Part model, mm, in its own coordinate system. A direction names the side the tool comes from. Round coordinates to 2 decimals unless told otherwise and drop trailing zeros. Order: outer loops, then holes, each group sorted by start corner. A loop starts at its lowest first (then second) coordinate and runs counter-clockwise, first axis right, second up. Notation, with made-up numbers: (61.25, -32.5) -> (93.25, -32.5) arc R22 ccw to (93.25, -19.5) -> close; hole circle Ø7 at (15, 71). An arc over 180 degrees is marked (long way). Answer as a JSON object with one key per item and string values. Group by question number.
```python
from build123d import *

# Parameters (mm, degrees)
SKETCH_W        = 120
SKETCH_H        = 100
PAD_DEPTH       = 22
SKETCH001_R     = 4.5
POCKET_DEPTH    = 22.001
POCKET001_DEPTH = 22.001
SKETCH003_R     = 1
POCKET002_DEPTH = 22.001
SKETCH004_R     = 10
POCKET003_DEPTH = 1.2
SKETCH005_R     = 3.25
POCKET004_DEPTH = 20.801
CHAMFER_SIZE    = 2.25


with BuildPart() as part:
    # Sketch → Pad (new body)
    with BuildSketch(Plane.XY):
        Rectangle(SKETCH_W, SKETCH_H)
    extrude(amount=PAD_DEPTH)

    # Sketch001 → Pocket (cut, through all)
    with BuildSketch(Plane(origin=(0, 0, 0), x_dir=(1, 0, 0), z_dir=(0, 0, -1))):
        with Locations((-49.725, 7.03)):
            Circle(SKETCH001_R)
        with Locations((0, -28.025)):
            Circle(SKETCH001_R)
        with Locations((49.725, 7.03)):
            Circle(SKETCH001_R)
    extrude(amount=-POCKET_DEPTH, mode=Mode.SUBTRACT)

    # Sketch002 → Pocket001 (cut, through all)
    with BuildSketch(Plane.XY.offset(22)):
        with BuildLine():
            Line((-60, -50), (-60, -36.5))
            Line((-60, -36.5), (-31, -36.5))
            ThreePointArc((-27, -40.5), (-28.171573, -37.671573), (-31, -36.5))
            Line((-27, -50), (-27, -40.5))
            Line((-27, -50), (-60, -50))
        make_face()
        with BuildLine():
            Line((60, -36.5), (60, -50))
            Line((60, -50), (27, -50))
            Line((27, -50), (27, -40.500015))
            ThreePointArc((31, -36.5), (28.171568, -37.671578), (27, -40.500015))
            Line((60, -36.5), (31, -36.5))
        make_face()
        with BuildLine():
            Line((13, 50), (-13, 50))
            Line((-13, 40.5), (-13, 50))
            ThreePointArc((-13, 40.5), (-11.828427, 37.671573), (-9, 36.5))
            Line((-9, 36.5), (9, 36.5))
            ThreePointArc((9, 36.5), (11.828427, 37.671573), (13, 40.5))
            Line((13, 40.5), (13, 50))
        make_face()
    extrude(amount=-POCKET001_DEPTH, mode=Mode.SUBTRACT)

    # Sketch003 → Pocket002 (cut, through all)
    with BuildSketch(Plane.XY.offset(22)):
        with Locations((50, -26.5)):
            Circle(SKETCH003_R)
        with Locations((-50, -26.5)):
            Circle(SKETCH003_R)
        with Locations((50, 40)):
            Circle(SKETCH003_R)
        with Locations((-50, 40)):
            Circle(SKETCH003_R)
    extrude(amount=-POCKET002_DEPTH, mode=Mode.SUBTRACT)

    # Sketch004 → Pocket003 (cut)
    with BuildSketch(Plane(origin=(0, 0, 0), x_dir=(1, 0, 0), z_dir=(0, 0, -1))):
        with Locations((0, 25)):
            Circle(SKETCH004_R)
        with Locations((-36, -25)):
            Circle(SKETCH004_R)
        with Locations((36, -25)):
            Circle(SKETCH004_R)
    extrude(amount=-POCKET003_DEPTH, mode=Mode.SUBTRACT)

    # Sketch005 → Pocket004 (cut, through all)
    with BuildSketch(Plane(origin=(0, 0, 1.2), x_dir=(1, 0, 0), z_dir=(0, 0, -1))):
        with Locations((0, 25)):
            Circle(SKETCH005_R)
        with Locations((36, -25)):
            Circle(SKETCH005_R)
        with Locations((-36, -25)):
            Circle(SKETCH005_R)
    extrude(amount=-POCKET004_DEPTH, mode=Mode.SUBTRACT)

    # Chamfer
    chamfer_edges = [part.edges().sort_by_distance(p)[0] for p in [
        (49, 40, 22),
        (49, -26.5, 22),
        (-51, -26.5, 22),
        (-51, 40, 22),
    ]]
    chamfer(chamfer_edges, length=CHAMFER_SIZE)


solid = part.part
```
Q1. Drop flat-ended pins along their axis: pin 1 Ø6.5 at (x, z) = (44, 6) entering from -Y; pin 2 Ø3 at (y, z) = (-43.5, 10.5) entering from +X. Give the stop position or say it passes through.
Q2. Two-plate mould, pull along Y, no slides. Class faces 1 (the flat face through (-37, 50, 11)), 2 (the flat face through (27, -45, 11)), 3 (the cylindrical face through (45.23, -7.23, 10.85)): +Y half, -Y half, draft (parallel to the pull), parting line (faces both ways), or undercut.
Q3. Which spindle directions (+Z, -Z, +X, -X, +Y, -Y) get a long thin tool onto all of the face, cutting with end or side? Do faces 4 (the flat face through (-46, -36.5, 11)), 5 (the cylindrical face through (-43.37, 18.24, 0.59)), 6 (the flat face through (0, 36.5, 11)), 7 (the flat face through (60, 6, 11)), 8 (the conical face through (51.025, -26.925, 19.859)). Say none if no direction does.
Q4. Band-saw the part on B-B (x = -36). List the corners of the cut face in (y, z), plus the area to 3 significant figures.
Q5. Band-saw the part on A-A (y = -7.03). List the corners of the cut face in (x, z) (3 decimals), plus the area to 3 significant figures.
Q6. Band-saw the part on D-D (z = 10.25). Count the separate pieces of the cut face and the enclosed holes in it, plus the area to 3 significant figures.
Q7. Band-saw the part on C-C (y = 25). List the corners of the cut face in (x, z), plus the area to 3 significant figures.
Q8. Wall check: line 1 (Y direction, x = 50, z = 5.5); line 2 (X direction, y = -7.03, z = 15.5) (3 decimals); line 3 (Y direction, x = 0, z = 0.35) (3 decimals). Give the ranges that are in metal, low to high. Write a range as [from, to].
Completed:
{
 "1": {"pin 1": "y = -36.5", "pin 2": "x = 27"},
 "2": {"face 1": "+Y half", "face 2": "draft", "face 3": "undercut"},
 "3": {"face 4": "+Z, -Z, -X, -Y", "face 5": "-Z", "face 6": "+Z, -Z, +Y", "face 7": "+Z, -Z, +X, +Y, -Y", "face 8": "+Z"},
 "4": {"outline": "(-36.5, 0) -> (15, 0) -> (15, 1.2) -> (21.75, 1.2) -> (21.75, 22) -> (-36.5, 22) -> close; (28.25, 1.2) -> (35, 1.2) -> (35, 0) -> (50, 0) -> (50, 22) -> (28.25, 22) -> close", "area": "1,740 mm2"},
 "5": {"outline": "(-60, 0) -> (-54.225, 0) -> (-54.225, 22) -> (-60, 22) -> close; (-45.225, 0) -> (45.225, 0) -> (45.225, 22) -> (-45.225, 22) -> close; (54.225, 0) -> (60, 0) -> (60, 22) -> (54.225, 22) -> close", "area": "2,240 mm2"},
 "6": {"separate pieces": "1", "enclosed holes": "10", "area": "10,500 mm2"},
 "7": {"outline": "(-60, 0) -> (-46, 0) -> (-46, 1.2) -> (-39.25, 1.2) -> (-39.25, 22) -> (-60, 22) -> close; (-32.75, 1.2) -> (-26, 1.2) -> (-26, 0) -> (-3.33, 0) -> (-3.33, 22) -> (-32.75, 22) -> close; (3.33, 0) -> (26, 0) -> (26, 1.2) -> (32.75, 1.2) -> (32.75, 22) -> (3.33, 22) -> close; (39.25, 1.2) -> (46, 1.2) -> (46, 0) -> (60, 0) -> (60, 22) -> (39.25, 22) -> close", "area": "2,180 mm2"},
 "8": {"line 1": "[-36.5, -27.5], [-25.5, -11.52], [-2.54, 39], [41, 50]", "line 2": "[-60, -54.225], [-45.225, 45.225], [54.225, 60]", "line 3": "[-50, -35], [-15, 23.525], [32.525, 36.5]"}
}
